Check sheet for the modelled part. Datum: model origin and axes. Units: mm. Face numbers are marked on the shaded views. Coordinates: 2 decimals unless noted, no trailing zeros. Loops run counter-clockwise (first coordinate to the right, second up) from the corner with the lowest first, then second, coordinate; pieces in that order, holes last. Notation, with made-up numbers: (59.5, 59) - (77.5, 59) arc R23 ccw to (77.5, 74) - close; hole circle Ø4 at (87.5, 9). An arc over 180 degrees is marked (long way). Write each question's results on one line, items separated by ' | '. Start each with the question number.
1. Cross-section at A-A (y = 0). Record the cut outline in (x, z).
2. Thickness scan on line 1 (Y direction, x = -0.5, z = 1.5); line 2 (X direction, y = 0, z = 3.75); line 3 (Z direction, x = 0, y = 15.3). Record the ranges inside material, lowest first. Write a range as [from, to].
3. Cross-section at D-D (x = -9). Record the cut outline in (y, z).
4. Gauge pin test, flat ends, axial feed: P1, Ø1.2, axis at x = 0, z = 5.08, coming from the -Y side; P2, Ø3, axis at x = -8, z = 5.5, coming from the -Y side; P3, Ø2, axis at x = -10.5, z = 1.5, coming from the +Y side; P4, Ø2, axis at x = -8.5, z = 6, coming from the -Y side. Record the tip position at first contact, or that the pin passes through.
5. Draft check along X on the marked faces 1, 2 and 3. Enter one of: released by +X, released by -X, zero draft, split by the parting line, or undercut.
6. Cross-section at C-C (y = -8). Record the cut outline in (x, z), and give its area (3 significant figures).
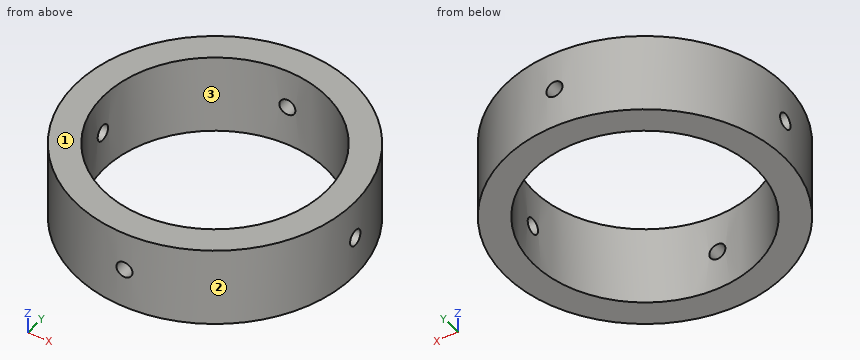
Autodesk Fusion 360 part; units mm, degrees
sketch "Sketch1" plane through (0, 0, 0) normal (0, 0, 1) x (1, 0, 0)
  circle A0 centre (0, 0) radius 14
  circle A1 centre (0, 0) radius 17.5
  dimension "d1" = 35
  dimension "d2" = 28
extrude "Extrude1" add sketch "Sketch1" along normal blind 10
sketch "Sketch2" plane through (0, 0, 0) normal (0, 1, 0) x (1, 0, 0)
  circle A0 centre (0, -5.08) radius 1
  dimension "d5" = 2
  dimension "d6" = 5.08
extrude "Extrude2" cut sketch "Sketch2" along normal through all and the other way through all
sketch "Sketch3" plane through (0, 0, 0) normal (1, 0, 0) x (0, 0, -1)
  circle A0 centre (-5.08, 0) radius 1
  dimension "d9" = 2
  dimension "d10" = 5.08
extrude "Extrude3" cut sketch "Sketch3" along normal through all and the other way through all
Established:
1) outline: (-17.5, 0) - (-14, 0) - (-14, 4.08) - (-17.5, 4.08) - close; (-17.5, 6.08) - (-14, 6.08) - (-14, 10) - (-17.5, 10) - close; (14, 0) - (17.5, 0) - (17.5, 4.08) - (14, 4.08) - close; (14, 6.08) - (17.5, 6.08) - (17.5, 10) - (14, 10) - close
2) line 1: [-17.49, -13.99], [13.99, 17.49] | line 2: [-17.5, -14], [14, 17.5] | line 3: [0, 4.08], [6.08, 10]
3) outline: (-15.01, 0) - (-10.72, 0) - (-10.72, 10) - (-15.01, 10) - close; (10.72, 0) - (15.01, 0) - (15.01, 10) - (10.72, 10) - close
4) P1: through | P2: y = -16.25 | P3: y = 14.7 | P4: y = -15.81
5) face 1: zero draft | face 2: split by the parting line | face 3: undercut
6) outline: (-15.56, 0) - (-11.49, 0) - (-11.49, 10) - (-15.56, 10) - close; (11.49, 0) - (15.56, 0) - (15.56, 10) - (11.49, 10) - close | area: 81.5 mm^2
